The listing builds one solid part. Answer for the finished solid, in the listing's coordinates (mm). Give positions to 0.01 mm unless a question says otherwise; leave off trailing zeros. Write each loop counter-clockwise with the first axis right and the second up, starting at its lowest first coordinate (ties: lowest second). Pieces come first, ordered by that corner, then holes. Notation, with made-up numbers: (47.25, 42.5) -> (77.25, 42.5) arc R19 cw to (77.25, 53.5) -> close; hole circle Ø10 at (2.25, 80.5). An arc over 180 degrees is marked (long way). Put each result on its own line as item: value. Start each with the question number.
1) A cutting plane is placed at A-A (x = 77). Write down the section's boundary in (y, z).
2) A cutting plane is placed at B-B (z = -77). Write down the section's boundary in (x, y).
3) Find the intervals of material crossed by line 1 along X through (y, z) = (6.75, -77); line 2 along Z through (x, y) = (77, 7); line 3 along X through (y, z) = (3, -33), in increasing order. Write a range as from..to.
4) For a pull along X with two mould halves and no side action, classify faces 1 (the cylindrical face through (34.72, 4.93, -123.03)), 2 (the flat face through (0, 5, -76)), 3 (the flat face through (76, 5, -154)), 4 (the flat face through (154, 5, -76)) as released by +X, released by -X, zero draft, split by the parting line, or undercut.
from build123d import *

# Parameters (mm, degrees)
SKETCH1_W           = 154
SKETCH1_H           = 154
BOSS_EXTRUDE1_DEPTH = 10


with BuildPart() as part:
    # Sketch1 → Boss-Extrude1 (new body)
    with BuildSketch(Plane(origin=(0, 0, 0), x_dir=(1, 0, 0), z_dir=(0, 1, 0))):
        with Locations((77, 77)):
            Rectangle(SKETCH1_W, SKETCH1_H)
        with BuildLine():
            ThreePointArc((125.861682212, 38.028394806), (32.805826176, 121.194173824), (115.971605194, 28.138317788))
            add(Edge.make_bspline(
                [(115.971605194, 28.138317788), (122.387611631, 21.271341921), (127.558134855, 26.441865145), (132.728658079, 31.612388369), (125.861682212, 38.028394806)],
                knots=[1.527172841, 1.527172841, 1.527172841, 3.141592654, 3.141592654, 4.756012466, 4.756012466, 4.756012466], degree=2, weights=[1, 0.691516576, 1, 0.691516576, 1]))
        make_face(mode=Mode.SUBTRACT)
    extrude(amount=BOSS_EXTRUDE1_DEPTH)


solid = part.part
Reply:
1. outline: (0, -154) -> (10, -154) -> (10, -139.5) -> (0, -139.5) -> close; (0, -14.5) -> (10, -14.5) -> (10, 0) -> (0, 0) -> close
2. outline: (0, 0) -> (14.5, 0) -> (14.5, 10) -> (0, 10) -> close; (139.5, 0) -> (154, 0) -> (154, 10) -> (139.5, 10) -> close
3. line 1: x = 0..14.5, 139.5..154
3. line 2: z = -154..-139.5, -14.5..0
3. line 3: x = 0..32.61, 128.96..154
4. face 1: undercut
4. face 2: released by -X
4. face 3: zero draft
4. face 4: released by +X
